Here's how the part is built. I have some questions about the finished solid (model axes, mm). A direction names the side the tool comes from. Round coordinates to 2 decimals unless told otherwise and drop trailing zeros. Loops run counter-clockwise (first coordinate to the right, second up) from the corner with the lowest first, then second, coordinate; pieces in that order, holes last. Notation, with made-up numbers: M -17.75,21.5 L -6.75,21.5 A23 cw -6.75,50.5 Z; hole C -6.5,2.25 d10. An arc over 180 degrees is marked long. Answer as a JSON object with one key per item and string values.
from build123d import *

# Parameters (mm, degrees)
F0_R     = 12.85
F1_DEPTH = 2
F3_DEPTH = 20
F4_R     = 1
F5_R     = 1.99999


# Not quite as in the source:
# - a fillet or chamfer is up to 0.001 mm smaller than in the source, because OpenCascade refuses the exact size


with BuildPart() as f1:
    # F0 (on Top) → F1 (new body)
    with BuildSketch(Plane.XY):
        Circle(F0_R)
    extrude(amount=F1_DEPTH)

    # F2 (on face) → F3 (join)
    with BuildSketch(Plane.XY.offset(2)):
        with BuildLine():
            ThreePointArc((11.4891252931, -0.5), (11.4972810018, -0.2500591226), (11.5, 0))
            ThreePointArc((11.5, 0), (11.4972810018, 0.2500591226), (11.4891252931, 0.5))
            Line((11.4891252931, 0.5), (9.9874921777, 0.5))
            ThreePointArc((9.9874921777, 0.5), (9.9968725554, 0.2500782106), (10, 0))
            ThreePointArc((10, 0), (9.9968725554, -0.2500782106), (9.9874921777, -0.5))
            Line((9.9874921777, -0.5), (11.4891252931, -0.5))
        make_face()
        with BuildLine():
            ThreePointArc((11.4891252931, 0.5), (11.4972810018, 0.2500591226), (11.5, 0))
            ThreePointArc((11.5, 0), (11.4972810018, -0.2500591226), (11.4891252931, -0.5))
            Line((11.4891252931, -0.5), (11.85, -0.5))
            Line((11.85, -0.5), (11.85, 0.5))
            Line((11.85, 0.5), (11.4891252931, 0.5))
        make_face()
        with BuildLine():
            Line((9.9874921777, 0.5), (11.4891252931, 0.5))
            ThreePointArc((11.4891252931, 0.5), (8.1317279836, 8.1317279836), (0.5, 11.4891252931))
            Line((0.5, 11.4891252931), (0.5, 9.9874921777))
            ThreePointArc((0.5, 9.9874921777), (7.0710678119, 7.0710678119), (9.9874921777, 0.5))
        make_face()
        with BuildLine():
            ThreePointArc((0.5, -11.4891252931), (8.1317279836, -8.1317279836), (11.4891252931, -0.5))
            Line((11.4891252931, -0.5), (9.9874921777, -0.5))
            ThreePointArc((9.9874921777, -0.5), (7.0710678119, -7.0710678119), (0.5, -9.9874921777))
            Line((0.5, -9.9874921777), (0.5, -11.4891252931))
        make_face()
        with BuildLine():
            Line((0.5, 9.9874921777), (0.5, 11.4891252931))
            ThreePointArc((0.5, 11.4891252931), (0, 11.5), (-0.5, 11.4891252931))
            Line((-0.5, 11.4891252931), (-0.5, 9.9874921777))
            ThreePointArc((-0.5, 9.9874921777), (0, 10), (0.5, 9.9874921777))
        make_face()
        with BuildLine():
            ThreePointArc((-0.5, 11.4891252931), (0, 11.5), (0.5, 11.4891252931))
            Line((0.5, 11.4891252931), (0.5, 11.85))
            Line((0.5, 11.85), (-0.5, 11.85))
            Line((-0.5, 11.85), (-0.5, 11.4891252931))
        make_face()
        with BuildLine():
            Line((0.5, -11.85), (0.5, -11.4891252931))
            ThreePointArc((0.5, -11.4891252931), (0, -11.5), (-0.5, -11.4891252931))
            Line((-0.5, -11.4891252931), (-0.5, -11.85))
            Line((-0.5, -11.85), (0.5, -11.85))
        make_face()
        with BuildLine():
            ThreePointArc((-0.5, -11.4891252931), (0, -11.5), (0.5, -11.4891252931))
            Line((0.5, -11.4891252931), (0.5, -9.9874921777))
            ThreePointArc((0.5, -9.9874921777), (0, -10), (-0.5, -9.9874921777))
            Line((-0.5, -9.9874921777), (-0.5, -11.4891252931))
        make_face()
        with BuildLine():
            Line((-0.5, 9.9874921777), (-0.5, 11.4891252931))
            ThreePointArc((-0.5, 11.4891252931), (-8.1317279836, 8.1317279836), (-11.4891252931, 0.5))
            Line((-11.4891252931, 0.5), (-9.9874921777, 0.5))
            ThreePointArc((-9.9874921777, 0.5), (-7.0710678119, 7.0710678119), (-0.5, 9.9874921777))
        make_face()
        with BuildLine():
            ThreePointArc((-11.4891252931, -0.5), (-8.1317279836, -8.1317279836), (-0.5, -11.4891252931))
            Line((-0.5, -11.4891252931), (-0.5, -9.9874921777))
            ThreePointArc((-0.5, -9.9874921777), (-7.0710678119, -7.0710678119), (-9.9874921777, -0.5))
            Line((-9.9874921777, -0.5), (-11.4891252931, -0.5))
        make_face()
        with BuildLine():
            Line((-9.9874921777, 0.5), (-11.4891252931, 0.5))
            ThreePointArc((-11.4891252931, 0.5), (-11.5, 0), (-11.4891252931, -0.5))
            Line((-11.4891252931, -0.5), (-9.9874921777, -0.5))
            ThreePointArc((-9.9874921777, -0.5), (-10, 0), (-9.9874921777, 0.5))
        make_face()
        with BuildLine():
            ThreePointArc((-11.4891252931, -0.5), (-11.5, 0), (-11.4891252931, 0.5))
            Line((-11.4891252931, 0.5), (-11.85, 0.5))
            Line((-11.85, 0.5), (-11.85, -0.5))
            Line((-11.85, -0.5), (-11.4891252931, -0.5))
        make_face()
    extrude(amount=F3_DEPTH)

    # F4
    f4_edges = [f1.edges().sort_by_distance(p)[0] for p in [
        (11.85, 0, 22),
        (0, 11.85, 22),
        (-11.85, 0, 22),
        (0, -11.85, 22),
    ]]
    fillet(f4_edges, radius=F4_R)

    # F5 (radius 2 in the source; OpenCascade refuses exactly that, so slightly less here)
    f5_edges = [f1.edges().sort_by_distance(p)[0] for p in [
        (-12.85, 0, 0),
    ]]
    fillet(f5_edges, radius=F5_R)


solid = f1.part
Item 1: I want a section at A-A, the plane z = 14. Please give me the cut outline in (x, y), then the cut area to 3 significant figures.
Resolved:
{"outline": "M -11.85,-0.5 L -11.49,-0.5 A11.5 ccw -0.5,-11.49 L -0.5,-11.85 L 0.5,-11.85 L 0.5,-11.49 A11.5 ccw 11.49,-0.5 L 11.85,-0.5 L 11.85,0.5 L 11.49,0.5 A11.5 ccw 0.5,11.49 L 0.5,11.85 L -0.5,11.85 L -0.5,11.49 A11.5 ccw -11.49,0.5 L -11.85,0.5 Z; hole C 0,0 d20", "area": "103 mm²"}
Item 2: I'm going to push flat-ended pins straight in: pin 1 Ø4 at (y, z) = (3, 9.5) entering from +X; pin 2 Ø10 at (x, z) = (1, 9) entering from +Y; pin 3 Ø0.8 at (x, z) = (0, 11.5) entering from -Y. Where does each tip first touch, or does it pass through?
Resolved:
{"pin 1": "x = 11.46", "pin 2": "y = 11.85", "pin 3": "y = -11.85"}
Item 3: On a 3-axis mill with a long thin cutter (end or side, diameter ignored), from which of +Z, -Z, +X, -X, +Y, -Y can I reach the whole of each face in a straight line? I mean faces 1 (the face through (8.047, -8.216, 11.86)), 2 (the face through (-8.047, 8.216, 11.86)), 3 (the face through (8.216, 8.047, 11.86)). Say none if no direction works.
Resolved:
{"face 1": "+Z, +X, -Y", "face 2": "+Z, -X, +Y", "face 3": "+Z, +X, +Y"}
Item 4: If we mould it in two halves opening along X, with no side actions, what happens to faces 4 (the face through (11.85, 0, 11)), 5 (the face through (0, -11.85, 11)), 6 (the face through (0, 0, 2)), 7 (the face through (-8.216, -8.047, 11.86))? For each: pulls with the +X half, pulls with the -X half, needs draft (parallel to the pull), parting line crosses it, or undercut.
Resolved:
{"face 4": "pulls with the +X half", "face 5": "needs draft", "face 6": "undercut", "face 7": "pulls with the -X half"}
Item 5: Please list where these lines run through material, in increasing order: probe 1 along Y at (x, z) = (0.25, 19); probe 2 along Z at (x, y) = (-6, 6.75); probe 3 along Y at (x, z) = (-6, 12.75). Write a range as from..to.
Resolved:
{"probe 1": "-11.85..-10, 10..11.85", "probe 2": "0..2", "probe 3": "-9.81..-8, 8..9.81"}
